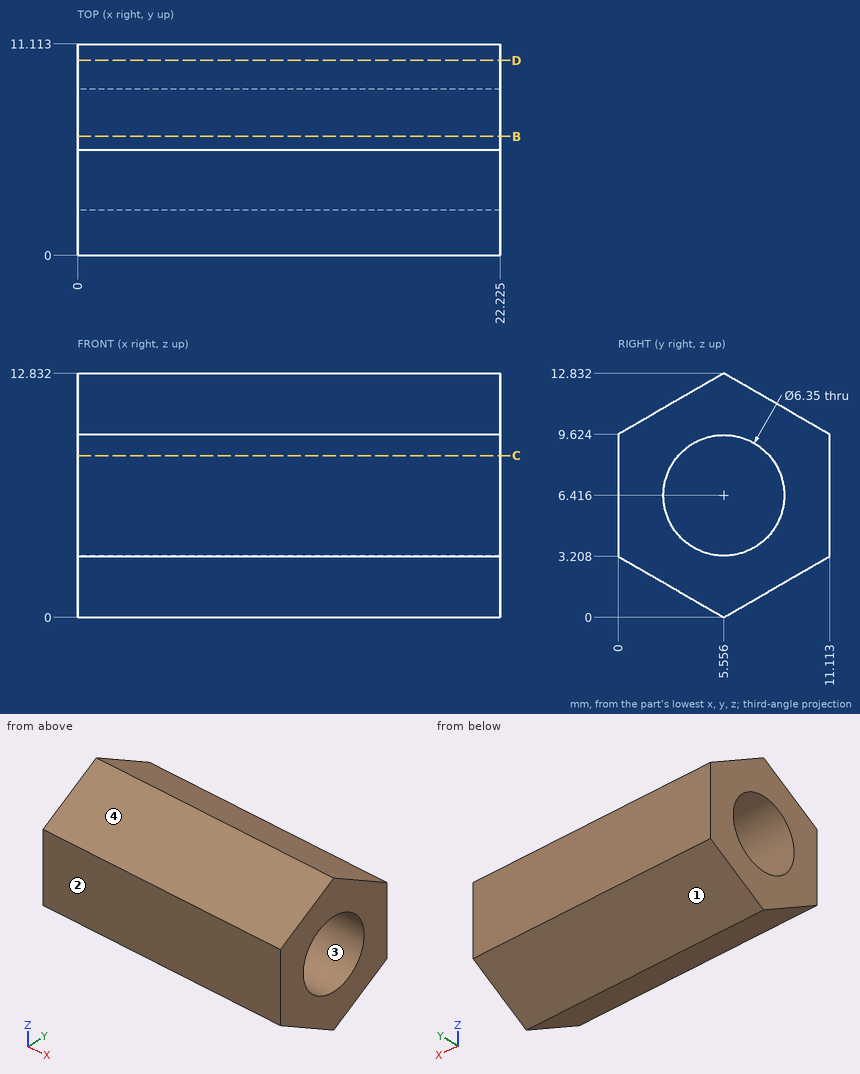
Print and shaded views of the part. All mm, measured from the part's lowest x, y and z. Give positions to 0.01 mm unless a question says otherwise; leave off trailing zeros. Loops run counter-clockwise (first coordinate to the right, second up) from the corner with the lowest first, then second, coordinate; pieces in that order, holes last. Notation, with made-up numbers: (8, 65) -> (43, 65) arc R10 cw to (43, 79) -> close; hole circle Ø5 at (37, -37.75). An arc over 180 degrees is marked (long way). Use CSV: the item, a comma, the result in double quotes. Start each with the question number.
1) Flat gauge pins, fed straight in: pin 1 Ø3 at (x, y) = (10, 8.5) entering from -Z; pin 2 Ø5.5 at (y, z) = (5.56, 6.42) entering from -X; pin 3 Ø4 at (x, y) = (3.5, 8.5) entering from +Z; pin 4 Ø1 at (x, z) = (12, 10.5) entering from -Y. Where does each tip first touch, or does it go through?
2) Wall check: line 1 (Y direction, x = 6.5, z = 6.5); line 2 (Z direction, x = 20.5, y = 4.25) (1 decimal); line 3 (Y direction, x = 20.25, z = 4) (1 decimal). Give the ranges that are in metal, low to high.
3) Slice it at D-D on y = 10.25. Give the cut face in (x, z) (1 decimal).
4) Slice it at B-B on y = 6.25. Give the cut face in (x, z) (1 decimal).
5) Mould opens along Z. For the marked faces 1, 2, 3 and 4 say: released by +Z, released by -Z, zero draft, split by the parting line, or undercut.
6) Slice it at C-C on z = 8.5. Give the cut face in (x, y) (1 decimal).
Computed values:
1,pin 1,"stops at z = 0.83"
1,pin 2,"passes through"
1,pin 3,"stops at z = 12.29"
1,pin 4,"stops at y = 0.65"
2,line 1,"y = 0 to 2.38, 8.73 to 11.11"
2,line 2,"z = 0.8 to 3.5, 9.3 to 12.1"
2,line 3,"y = 0 to 3.5, 7.6 to 11.1"
3,outline,"(0, 2.7) -> (22.2, 2.7) -> (22.2, 10.1) -> (0, 10.1) -> close"
4,outline,"(0, 0.4) -> (22.2, 0.4) -> (22.2, 3.3) -> (0, 3.3) -> close; (0, 9.5) -> (22.2, 9.5) -> (22.2, 12.4) -> (0, 12.4) -> close"
5,face 1,"released by -Z"
5,face 2,"zero draft"
5,face 3,"undercut"
5,face 4,"released by +Z"
6,outline,"(0, 0) -> (22.2, 0) -> (22.2, 3.2) -> (0, 3.2) -> close; (0, 8) -> (22.2, 8) -> (22.2, 11.1) -> (0, 11.1) -> close"
